For this review, take the finished solid that the model builds, in its own axes (mm). A direction names the side the tool comes from. Coordinates: 2 decimals unless noted, no trailing zeros. Write each loop counter-clockwise with the first axis right and the second up, starting at its lowest first coordinate (ties: lowest second). Pieces come first, ordered by that corner, then holes. Notation, with made-up numbers: M -10,89.5 L 34,89.5 A16 cw 34,113.5 Z; hole C 35.25,21 d1. An arc over 180 degrees is marked long. One line per question, with ' | ' between items.
from build123d import *
from build123d.topology import SkipClean

# Parameters (mm, degrees)
SKETCH1_R                 = 1.55
BOSS_EXTRUDE1_DEPTH       = 5
BOSS_EXTRUDE2_START       = 2
SKETCH2_R                 = 1.55
BOSS_EXTRUDE2_DEPTH       = 2
CHAMFER1_SIZE2            = 2
CHAMFER1_SIZE             = 3
BOSS_EXTRUDE3_START       = 18.1
SKETCH3_W                 = 10
SKETCH3_H                 = 8
SKETCH3_R                 = 1.55
BOSS_EXTRUDE3_DEPTH       = 18.1
BOSS_EXTRUDE4_DEPTH       = 10
CHAMFER2_SIZE             = 10
SKETCH6_R                 = 2.25
CUT_EXTRUDE2_DEPTH        = 81.396579529
SKETCH7_R                 = 3.5
CUT_EXTRUDE3_DEPTH        = 3
CHAMFER3_SIZE2            = 1.25
CHAMFER3_SIZE             = 2.5
CHAMFER3_OF_MIRROR2_SIZE2 = 1.25
CHAMFER3_OF_MIRROR2_SIZE  = 2.5


with BuildPart() as part:
    # Sketch1 → Boss-Extrude1 (new body)
    with BuildSketch(Plane(origin=(0, 0, 0), x_dir=(1, 0, 0), z_dir=(0, 1, 0))):
        with BuildLine():
            Line((0, 4), (-31, 4))
            Line((-31, 4), (-31, -4))
            Line((-31, -4), (0, -4))
            ThreePointArc((0, -4), (4, 0), (0, 4))
        make_face()
        with Locations(Location((0, 0, 0), (0, 0, 270))):
            Circle(SKETCH1_R, mode=Mode.SUBTRACT)
        with Locations(Location((-26, 0, 0), (0, 0, 270))):
            Circle(SKETCH1_R, mode=Mode.SUBTRACT)
    extrude(amount=BOSS_EXTRUDE1_DEPTH)

    # Sketch2 → Boss-Extrude2 (add)
    with SkipClean():  # the faces are left unmerged after this step: merging them gives an invalid solid
        with BuildSketch(Plane.XZ.offset(BOSS_EXTRUDE2_START)):
            with BuildLine():
                Line((0, 4), (-2.5, 4))
                Line((-2.5, 4), (-2.5, -4))
                Line((-2.5, -4), (0, -4))
                ThreePointArc((0, -4), (4, 0), (0, 4))
            make_face()
            with Locations(Location((0, 0, 0), (0, 0, 270))):
                Circle(SKETCH2_R, mode=Mode.SUBTRACT)
        extrude(amount=-BOSS_EXTRUDE2_DEPTH)

    # Chamfer1
    chamfer1_edges = [part.edges().sort_by_distance(p)[0] for p in [
        (-2.5, 0, 0),
    ]]
    chamfer1_side = [part.faces().sort_by_distance(p)[0] for p in [
        (-2.54, 0, 0),
    ]]
    chamfer(chamfer1_edges, length=CHAMFER1_SIZE - 0.0001, length2=CHAMFER1_SIZE2 - 0.0001, reference=chamfer1_side[0])  # a hair under: the kernel refuses the full size

    # Sketch3 → Boss-Extrude3 (add)
    with BuildSketch(Plane.XZ.offset(BOSS_EXTRUDE3_START)):
        with Locations((-26, 0)):
            Rectangle(SKETCH3_W, SKETCH3_H)
        with Locations(Location((-26, 0, 0), (0, 0, 270))):
            Circle(SKETCH3_R, mode=Mode.SUBTRACT)
    extrude(amount=-BOSS_EXTRUDE3_DEPTH)

    # Sketch4 → Boss-Extrude4 (add)
    with BuildSketch(Plane.ZY.offset(31)):
        Polygon((-4, -18.1), (-22, -18.1), (-25, -21.1), (-25, -62.1), (-39, -62.1), (-39, -58.1), (-29, -58.1), (-29, -20), (-4, 5), align=None)
    boss_extrude4 = extrude(amount=-BOSS_EXTRUDE4_DEPTH)

    # Mirror1: Boss-Extrude4 across plane
    add(boss_extrude4.mirror(Plane.XY))

    # Chamfer2
    chamfer2_edges = [part.edges().sort_by_distance(p)[0] for p in [
        (-21, 0, 0),
    ]]
    chamfer(chamfer2_edges, length=CHAMFER2_SIZE)

    # Sketch6 → Cut-Extrude2 (cut, through all)
    with BuildSketch(Plane(origin=(0, -58.1, 0), x_dir=(1, 0, 0), z_dir=(0, 1, 0))):
        with Locations(Location((-26, -34, 0), (0, 0, 270))):
            Circle(SKETCH6_R)
    cut_extrude2 = extrude(amount=-CUT_EXTRUDE2_DEPTH, mode=Mode.SUBTRACT)

    # Sketch7 → Cut-Extrude3 (cut)
    with BuildSketch(Plane(origin=(0, -58.1, 0), x_dir=(1, 0, 0), z_dir=(0, 1, 0))):
        with Locations(Location((-26, -34, 0), (0, 0, 270))):
            Circle(SKETCH7_R)
    cut_extrude3 = extrude(amount=-CUT_EXTRUDE3_DEPTH, mode=Mode.SUBTRACT)

    # Chamfer3
    chamfer3_edges = [part.edges().sort_by_distance(p)[0] for p in [
        (-26, -61.1, 30.5),
    ]]
    chamfer3_side = [part.faces().sort_by_distance(p)[0] for p in [
        (-26, -61.075, 30.5),
    ]]
    chamfer(chamfer3_edges, length=CHAMFER3_SIZE - 0.0001, length2=CHAMFER3_SIZE2 - 0.0001, reference=chamfer3_side[0])  # a hair under: the kernel refuses the full size

    # Mirror2: Cut-Extrude2, Cut-Extrude3 across plane
    add(cut_extrude2.mirror(Plane.XY), mode=Mode.SUBTRACT)
    add(cut_extrude3.mirror(Plane.XY), mode=Mode.SUBTRACT)

    # Chamfer3 of Mirror2
    chamfer3_of_mirror2_edges = [part.edges().sort_by_distance(p)[0] for p in [
        (-26, -61.1, -30.5),
    ]]
    chamfer3_of_mirror2_side = [part.faces().sort_by_distance(p)[0] for p in [
        (-26, -61.075, -30.5),
    ]]
    chamfer(chamfer3_of_mirror2_edges, length=CHAMFER3_OF_MIRROR2_SIZE - 0.0001, length2=CHAMFER3_OF_MIRROR2_SIZE2 - 0.0001, reference=chamfer3_of_mirror2_side[0])  # a hair under: the kernel refuses the full size


solid = part.part
1. Draft analysis for pull direction X (two halves, no side actions). For faces 1 (the flat face through (-4, -1, 0)), 2 (the flat face through (-26, -8, 17)), 3 (the flat face through (-21, -16, 3)), 4 (the flat face through (-31, -16, 3)), state which applies: pulls with the +X half, pulls with the -X half, needs draft (parallel to the pull), parting line crosses it, or undercut.
Computed values:
face 1: undercut | face 2: needs draft | face 3: pulls with the +X half | face 4: pulls with the -X half
2. Take a section at B-B on z = 0. Give the number of separate pieces and of enclosed holes in the cut face, plus the area to 3 significant figures.
Computed values:
separate pieces: 3 | enclosed holes: 0 | area: 329 mm2
3. For line 1 along X through (y, z) = (0.25, 0); line 2 along X through (y, z) = (-58.25, -34); line 3 along Y through (x, z) = (-26, 2.5), list the stretches that pass through material, from the lowest coordinate up.
Computed values:
line 1: x = -31 to -27.55, -24.45 to -1.55, 1.55 to 4 | line 2: x = -31 to -29.5, -22.5 to -21 | line 3: y = -18.1 to 5
4. Take a section at C-C on y = -25.5. State the section outline as (x, z) points, plus the area to 3 significant figures.
Computed values:
outline: M -31,-29 L -21,-29 L -21,-25 L -31,-25 Z; M -31,25 L -21,25 L -21,29 L -31,29 Z | area: 80.0 mm2
5. Take a section at D-D on y = -8.5. State the section outline as (x, z) points, plus the area to 3 significant figures.
Computed values:
outline: M -31,-17.5 L -21,-17.5 L -21,-4 L -19.5,-4 L -19.5,4 L -21,4 L -21,17.5 L -31,17.5 Z; hole C -26,0 d3.1 | area: 354 mm2
6. Machinability: for faces 5 (the flat face through (-26, -39, 29)), 6 (the flat face through (-13, 1, -4)), 7 (the cylindrical face through (-22.53, -58.35, -33.54)), 8 (the flat face through (-16, -5, 0)), 9 (the flat face through (1.43, -2, 0.94)), which of the approach directions +Z, -Z, +X, -X, +Y, -Y give a long, thin tool a straight path to every point of the face, cutting with its end or side? Answer none if there is none.
Computed values:
face 5: +Z, +X, -X, +Y | face 6: -Z, +X, +Y, -Y | face 7: +Y | face 8: +Z, -Z, -Y | face 9: +Z, -Z, +X, -Y
7. Clearance check with flat-ended pins moving along their axes: P1, Ø2, axis at x = -22, y = -36.5, coming from the -Z side; P2, Ø4.5, axis at x = -14, y = 0.5, coming from the +Z side; P3, Ø5, axis at x = -25, y = -33.5, coming from the +Z side. State where each tip first meets the part, or that it passes through.
Computed values:
P1: stops at z = -29 | P2: stops at z = 4 | P3: stops at z = 29
